Job drawing, mm, ordinate dimensions from the low corner. One solid piece. A direction names the side the tool comes from. Round coordinates to 2 decimals unless told otherwise and drop trailing zeros. Order: outer loops, then holes, each group sorted by start corner. A loop starts at its lowest first (then second) coordinate and runs counter-clockwise, first axis right, second up. Notation, with made-up numbers: M -21,10.25 L 26,10.25 A11 cw 26,24.25 Z; hole C 88,68 d7. An arc over 180 degrees is marked long. Answer as a JSON object with one key per item and string values. Group by question number.
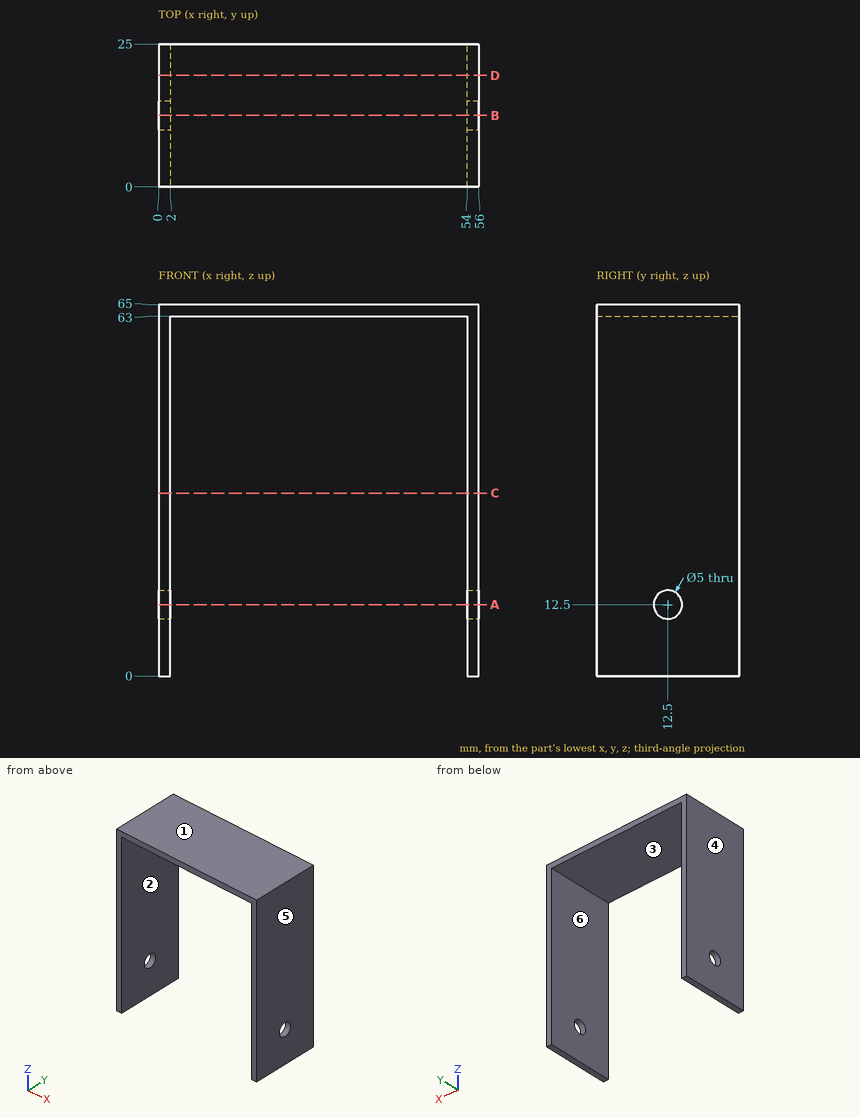
Item 1: Two-plate mould, pull along X, no slides. Class the marked faces 3, 4, 5 and 6: +X half, -X half, draft (parallel to the pull), parting line (faces both ways), or undercut.
Item 2: Flat gauge pins, fed straight in: pin 1 Ø8 at (x, y) = (23, 6.5) entering from -Z; pin 2 Ø1.5 at (y, z) = (11.5, 11) entering from -X; pin 3 Ø4.5 at (y, z) = (12.5, 12.5) entering from -X. Where does each tip first touch, or does it go through?
Item 3: Cut at C-C, the plane z = 32. Give the cut face in (x, y), and give its area (3 significant figures).
Item 4: Cut at A-A, the plane z = 12.5. Give the cut face in (x, y).
Item 5: Drill centre lines: line 1 (X direction, y = 15, z = 12); line 2 (Z direction, x = 55.1, y = 12.5); line 3 (Z direction, x = 53.5, y = 4.25). Where is each one in solid material? Low to high. Write a range as [from, to].
Item 6: Cut at D-D, the plane y = 19.5. Give the cut face in (x, z).
Item 7: Cut at B-B, the plane y = 12.5. Give the cut face in (x, z), and give its area (3 significant figures).
Item 8: 3-axis set-ups, long thin cutter, end or side, ignore diameter. For the marked faces 1 and 2: which of +Z, -Z, +X, -X, +Y, -Y reach the whole face in a straight line?
Response values:
{
 "1": {"face 3": "undercut", "face 4": "-X half", "face 5": "+X half", "face 6": "undercut"},
 "2": {"pin 1": "z = 63", "pin 2": "x = 0", "pin 3": "through"},
 "3": {"outline": "M 0,0 L 2,0 L 2,25 L 0,25 Z; M 54,0 L 56,0 L 56,25 L 54,25 Z", "area": "100 mm^2"},
 "4": {"outline": "M 0,0 L 2,0 L 2,10 L 0,10 Z; M 0,15 L 2,15 L 2,25 L 0,25 Z; M 54,0 L 56,0 L 56,10 L 54,10 Z; M 54,15 L 56,15 L 56,25 L 54,25 Z"},
 "5": {"line 1": "[0, 2], [54, 56]", "line 2": "[0, 10], [15, 65]", "line 3": "[63, 65]"},
 "6": {"outline": "M 0,0 L 2,0 L 2,63 L 54,63 L 54,0 L 56,0 L 56,65 L 0,65 Z"},
 "7": {"outline": "M 0,0 L 2,0 L 2,10 L 0,10 Z; M 0,15 L 2,15 L 2,63 L 54,63 L 54,15 L 56,15 L 56,65 L 0,65 Z; M 54,0 L 56,0 L 56,10 L 54,10 Z", "area": "344 mm^2"},
 "8": {"face 1": "+Z, +X, -X, +Y, -Y", "face 2": "-Z, +Y, -Y"}
}
